Design review of the part shown in the three views and the two pictorial views. Dimensions are in mm from the part's minimum x, y and z. Give positions to 0.01 mm unless a question says otherwise; leave off trailing zeros. Order: outer loops, then holes, each group sorted by start corner. A loop starts at its lowest first (then second) coordinate and runs counter-clockwise, first axis right, second up.
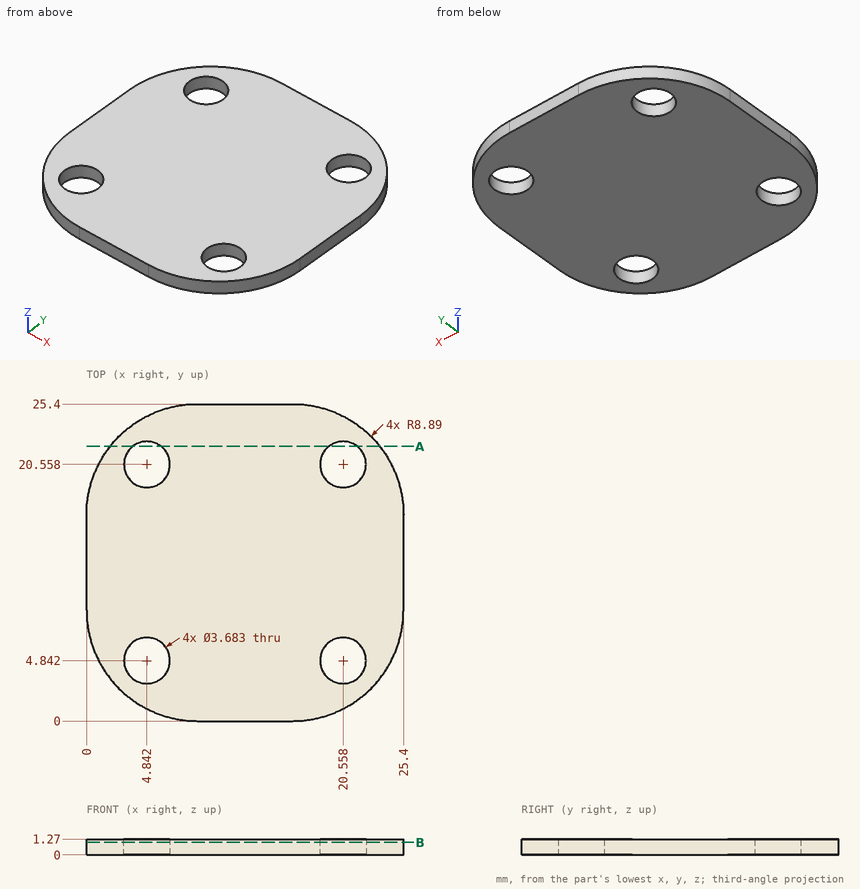
1) We need section A-A on y = 22. Give the boundary of the cut face in (x, z).
Answer sheet:
outline: (1.9, 0) - (3.7, 0) - (3.7, 1.27) - (1.9, 1.27) - close; (5.99, 0) - (19.41, 0) - (19.41, 1.27) - (5.99, 1.27) - close; (21.7, 0) - (23.5, 0) - (23.5, 1.27) - (21.7, 1.27) - close
2) Clearance check with a flat-ended pin moving along its axis: pin 1 (4 mm diameter, centred on x = 4.84, y = 4.84, fed in from +Z). State where the tip first meets the part, or that it passes through.
Answer sheet:
pin 1: stops at z = 1.27
3) We need section B-B on z = 1. Give the boundary of the cut face in (x, y).
Answer sheet:
outline: (0, 8.89) arc R8.89 ccw to (8.89, 0) - (16.51, 0) arc R8.89 ccw to (25.4, 8.89) - (25.4, 16.51) arc R8.89 ccw to (16.51, 25.4) - (8.89, 25.4) arc R8.89 ccw to (0, 16.51) - close; hole circle Ø3.68 at (4.84, 4.84); hole circle Ø3.68 at (4.84, 20.56); hole circle Ø3.68 at (20.56, 4.84); hole circle Ø3.68 at (20.56, 20.56)
4) To check wall thickness, follow line 1 (X direction, y = 20.5, z = 0.7) (1 decimal); line 2 (X direction, y = 19, z = 0.5) (1 decimal); line 3 (Y direction, x = 4.5, z = 1.1). State the ranges of each line that lie inside material, in increasing order.
Answer sheet:
line 1: x = 0.9 to 3, 6.7 to 18.7, 22.4 to 24.5
line 2: x = 0.4 to 3.9, 5.8 to 19.6, 21.5 to 25
line 3: y = 1.16 to 3.03, 6.65 to 18.75, 22.37 to 24.24
